Design review of the part built by this model. Coordinates are the model's own, in mm. A direction names the side the tool comes from. Round coordinates to 2 decimals unless told otherwise and drop trailing zeros. Write each loop counter-clockwise with the first axis right and the second up, starting at its lowest first coordinate (ties: lowest second). Pieces come first, ordered by that corner, then holes.
from build123d import *

# Parameters (mm, degrees)
F1_DEPTH        = 10
F5_R            = 2
F6_W            = 50
F6_H            = 45
F7_DEPTH        = 20
F10_D           = 2
F10_DEPTH       = 20
F10_CSINK_D     = 10
F10_CSINK_ANGLE = 82
F11_R           = 5
F12_R           = 1.75
F13_DEPTH       = 5


with BuildPart() as f1:
    # F0 (on Right) → F1 (new body, symmetric)
    with BuildSketch(Plane.YZ):
        with BuildLine():
            Line((-15, 0), (0, 0))
            Line((0, 0), (0, 24.5))
            Line((0, 24.5), (-5, 24.5))
            ThreePointArc((-5, 24.5), (-11.367509, 12.808167), (-15, 0))
        make_face()
    extrude(amount=F1_DEPTH, both=True)

    # F3 (on Right) → F4 (revolve)
    with BuildSketch(Plane.YZ):
        Polygon((0, 12.25), (15, 12.25), (15, 13.75), (10, 13.75), (1.75, 16.75), (1.75, 15.5), (0, 15.5), align=None)
    revolve(axis=Axis((0, 7.5, 12.25), (0, -1, 0)))

    # F5
    f5_edges = [f1.edges().sort_by_distance(p)[0] for p in [
        (0, -5, 24.5),
        (0, -15, 0),
        (0, 0, 0),
    ]]
    fillet(f5_edges, radius=F5_R)


with BuildPart() as f7:
    # F6 (on Right) → F7 (new body)
    with BuildSketch(Plane.YZ):
        with Locations((0, 10)):
            Rectangle(F6_W, F6_H)
    extrude(amount=F7_DEPTH)

    # F8: cut F1
    add(f1.part, mode=Mode.SUBTRACT)

    # F10
    with Locations(Plane.XZ.offset(25)):
        with Locations((0, 12.25)):
            CounterSinkHole(F10_D / 2, F10_CSINK_D / 2, depth=F10_DEPTH, counter_sink_angle=F10_CSINK_ANGLE)

    # F11
    f11_edges = [f7.edges().sort_by_distance(p)[0] for p in [
        (10, -25, 32.5),
        (10, 25, 32.5),
        (10, -25, -12.5),
        (10, 25, -12.5),
    ]]
    fillet(f11_edges, radius=F11_R)

    # F12 (on face) → F13 (join)
    with BuildSketch(Plane.YZ):
        with Locations((20, 27.5)):
            Circle(F12_R)
        with Locations((-20, 27.5)):
            Circle(F12_R)
        with Locations((-20, -7.5)):
            Circle(F12_R)
        with Locations((20, -7.5)):
            Circle(F12_R)
    extrude(amount=-F13_DEPTH)


solid = f7.part
1) Add section D-D on y = 7. State the section outline as (x, z) points, and give its area (3 significant figures).
2) Add section A-A on y = -3. State the section outline as (x, z) points.
3) Add section B-B on x = -1.5. State the section outline as (y, z) points, and give its area (3 significant figures).
4) For faces 4 (the face through (10, -25, 10)), 5 (the face through (-2.46, -21.39, -8.56)), list the 3-axis set-ups (+Z, -Z, +X, -X, +Y, -Y) from which the entire face can be reached by the end or side of a thin tool; tool diameter is ignored.
5) For P1, Ø10, axis at y = 11, z = 4, coming from the -X side; P2, Ø0.5, axis at x = 0.5, z = 12, coming from the -Y side, all flat-tipped, find the tip position at first contact; note any pin that passes through.
6) Add section C-C on z = -2. State the section outline as (x, y) points, and give its area (3 significant figures).
7) The part is to be moulded in two halves that separate along Z. For faces 1 (the face through (10, 0, 32.5)), 2 (the face through (10.14, 23.57, -11)), 3 (the face through (1, -15.7, 12.3)), say which applies: pulls with the +Z half, pulls with the -Z half, needs draft (parallel to the pull), parting line crosses it, or undercut.
8) For line 1 along X through (y, z) = (4, 18); line 2 along X through (y, z) = (-5, 23); line 3 along Y through (x, z) = (-1, 26), list the stretches that pass through material, from the lowest coordinate up.
Computed:
1. outline: (0, -12.5) - (20, -12.5) - (20, 32.5) - (0, 32.5) - (0, 14.84) arc R2.59 cw to (0, 9.66) - close
1. area: 889 mm2
2. outline: (0, -12.5) - (20, -12.5) - (20, 32.5) - (0, 32.5) - (0, 24.5) - (10, 24.5) - (10, 0) - (0, 0) - close
3. outline: circle Ø3.5 at (-20, -7.5); circle Ø3.5 at (-20, 27.5); circle Ø3.5 at (20, -7.5); circle Ø3.5 at (20, 27.5)
3. area: 38.5 mm2
4. face 4: +Z, -Z, +X, -X, -Y
4. face 5: -X
5. P1: stops at x = 0
5. P2: stops at y = 15
6. outline: (0, -25) - (20, -25) - (20, 25) - (0, 25) - close
6. area: 1,000 mm2
7. face 1: pulls with the +Z half
7. face 2: pulls with the -Z half
7. face 3: undercut
8. line 1: x = 0 to 20
8. line 2: x = 10 to 20
8. line 3: y = -20.9 to -19.1, 19.1 to 20.9
